Work out the finished part from the listing and answer in its coordinate system (mm). A direction names the side the tool comes from. Give positions to 0.01 mm unless a question says otherwise; leave off trailing zeros. Loops run counter-clockwise (first coordinate to the right, second up) from the corner with the lowest first, then second, coordinate; pieces in that order, holes last. Notation, with made-up numbers: M 5,82 L 54,82 A16 cw 54,94 Z; hole C 8.5,38.25 d6. An arc over 180 degrees is marked long. Write item = value, one per line. Start each with the question number.
1. Consider L1, parallel to X at y = 8.4, z = 25; L2, parallel to X at y = 5.25, z = -35.5; L3, parallel to Y at x = 48.5, z = -9.5. Determine where each line is inside the solid, lowest interval first. Write a range as [from, to].
2. Flat-ended cylindrical pins translate along their axes: pin 1 Ø0.6 at (x, z) = (0.5, -70) entering from +Y; pin 2 Ø1.5 at (x, z) = (-37, 10) entering from -Y; pin 3 Ø6 at (x, y) = (54.5, 0.5) entering from +Z; pin 4 Ø6 at (x, z) = (-55, 0) entering from +Y. Find the tip coordinate at first contact, or state that the pin passes through.
3. Section A-A on y = -5 is taken. Determine the outline of the cut face in (x, z), plus the area to 3 significant figures.
4. The mould has two halves that part along X. Classify faces 5 (the face through (-1, -6.3, -68.5)), 6 (the face through (-50.043, 7.535, -0.651)), 7 (the face through (1, -6.3, 68.6)): released by +X, released by -X, zero draft, split by the parting line, or undercut.
5. For faces 1 (the face through (1, -6.3, -68.5)), 2 (the face through (-1.915, 7.535, 50.669)), 3 (the face through (-1, 5, -1)), 4 (the face through (-1, -6.3, 68.6)), determine the directions among +Z, -Z, +X, -X, +Y, -Y from which every point of the face is accessible in a straight line to the end or side of a thin tool.
6. Section B-B on x = 20 is taken. Give the number of separate pieces and of enclosed holes in the cut face, plus the area to 3 significant figures.
7. Section C-C on y = 2.75 is taken. Determine the outline of the cut face in (x, z), plus the area to 3 significant figures.
```python
from build123d import *

# Parameters (mm, degrees)
SKETCH1_R           = 71.05
BOSS_EXTRUDE1_DEPTH = 10
BOSS_EXTRUDE1_TAPER = 5
SHELL4_T            = -5
SKETCH2_R           = 5
SKETCH2_R_2         = 25
SKETCH2_R_3         = 2.413
CUT_EXTRUDE1_DEPTH  = 101.976259737
CUT_EXTRUDE4_DEPTH  = 10
FILLET2_R           = 5
SKETCH11_R          = 5
CUT_EXTRUDE8_DEPTH  = 101.976259737
SKETCH12_W          = 2
SKETCH12_H          = 2
BOSS_EXTRUDE4_DEPTH = 7.5
SKETCH13_W          = 2
SKETCH13_H          = 4
BOSS_EXTRUDE5_DEPTH = 3
CUT_EXTRUDE9_DEPTH  = 3
CUT_EXTRUDE10_DEPTH = 3
CUT_EXTRUDE11_DEPTH = 3
CUT_EXTRUDE12_DEPTH = 3
CUT_EXTRUDE13_DEPTH = 3
CUT_EXTRUDE14_DEPTH = 3


with BuildPart() as part:
    # Sketch1 → Boss-Extrude1 (new body)
    with BuildSketch(Plane(origin=(0, 0, 0), x_dir=(1, 0, 0), z_dir=(0, 1, 0))):
        Circle(SKETCH1_R)
    extrude(amount=BOSS_EXTRUDE1_DEPTH, taper=BOSS_EXTRUDE1_TAPER)

    # Shell4
    shell4_openings = [part.faces().sort_by_distance(p)[0] for p in [
        (0, 0, 0),
    ]]
    offset(amount=SHELL4_T, openings=shell4_openings, kind=Kind.INTERSECTION)

    # Sketch2 → Cut-Extrude1 (cut, through all)
    with BuildSketch(Plane(origin=(0, 10, 0), x_dir=(1, 0, 0), z_dir=(0, 1, 0))):
        with Locations(Location((0, -46.05, 0), (0, 0, 270))):
            Circle(SKETCH2_R)
        with Locations(Location((0, 36.05, 0), (0, 0, 270))):
            Circle(SKETCH2_R_2)
        with Locations(Location((20, 5, 0), (0, 0, 270))):
            Circle(SKETCH2_R_3)
        with Locations(Location((20, -25, 0), (0, 0, 270))):
            Circle(SKETCH2_R_3)
        with Locations(Location((-20, -25, 0), (0, 0, 270))):
            Circle(SKETCH2_R_3)
        with Locations(Location((-20, 5, 0), (0, 0, 270))):
            Circle(SKETCH2_R_3)
    extrude(amount=-CUT_EXTRUDE1_DEPTH, mode=Mode.SUBTRACT)

    # Sketch6 → Cut-Extrude4 (cut)
    with BuildSketch(Plane(origin=(0, 10, 0), x_dir=(1, 0, 0), z_dir=(0, 1, 0))):
        with BuildLine():
            Line((-2.5, 14.187111582), (2.5, 14.187111582))
            Line((2.5, 14.187111582), (2.5, 9.55))
            ThreePointArc((2.5, 9.55), (2.207106781, 8.842893219), (1.5, 8.55))
            Line((1.5, 8.55), (-1.5, 8.55))
            ThreePointArc((-1.5, 8.55), (-2.207106781, 8.842893219), (-2.5, 9.55))
            Line((-2.5, 9.55), (-2.5, 14.187111582))
        make_face()
    extrude(amount=-CUT_EXTRUDE4_DEPTH, mode=Mode.SUBTRACT)

    # Fillet2
    fillet2_edges = [part.edges().sort_by_distance(p)[0] for p in [
        (-70.175113365, 10, 0),
    ]]
    fillet(fillet2_edges, radius=FILLET2_R)

    # Sketch11 → Cut-Extrude8 (cut, through all)
    with BuildSketch(Plane(origin=(0, 10, 0), x_dir=(1, 0, 0), z_dir=(0, 1, 0))):
        with Locations(Location((-55, 0, 0), (0, 0, 270))):
            Circle(SKETCH11_R)
    extrude(amount=-CUT_EXTRUDE8_DEPTH, mode=Mode.SUBTRACT)

    # Sketch12 → Boss-Extrude4 (add)
    with BuildSketch(Plane(origin=(0, 0, 0), x_dir=(-1, 0, 0), z_dir=(0, -1, 0))):
        Polygon((58.523702054, 32.633974596), (60.255752861, 33.633974596), (59.255752861, 35.366025404), (57.523702054, 34.366025404), align=None)
        with Locations((0, 68)):
            Rectangle(SKETCH12_W, SKETCH12_H)
        Polygon((57.523702054, -34.366025404), (59.255752861, -35.366025404), (60.255752861, -33.633974596), (58.523702054, -32.633974596), align=None)
        with Locations((0, -68)):
            Rectangle(SKETCH12_W, SKETCH12_H)
        Polygon((-58.523702054, -32.633974596), (-60.255752861, -33.633974596), (-59.255752861, -35.366025404), (-57.523702054, -34.366025404), align=None)
        Polygon((-57.523702054, 34.366025404), (-59.255752861, 35.366025404), (-60.255752861, 33.633974596), (-58.523702054, 32.633974596), align=None)
    extrude(amount=BOSS_EXTRUDE4_DEPTH)

    # Sketch13 → Boss-Extrude5 (add)
    with BuildSketch(Plane(origin=(0, -7.5, 0), x_dir=(-1, 0, 0), z_dir=(0, -1, 0))):
        Polygon((-58.523702054, -32.633974596), (-61.987803669, -34.633974596), (-60.987803669, -36.366025404), (-57.523702054, -34.366025404), align=None)
        with Locations((0, -69)):
            Rectangle(SKETCH13_W, SKETCH13_H)
        Polygon((-57.523702054, 34.366025404), (-60.987803669, 36.366025404), (-61.987803669, 34.633974596), (-58.523702054, 32.633974596), align=None)
        with Locations((0, 69)):
            Rectangle(SKETCH13_W, SKETCH13_H)
        Polygon((58.523702054, 32.633974596), (61.987803669, 34.633974596), (60.987803669, 36.366025404), (57.523702054, 34.366025404), align=None)
        Polygon((57.523702054, -34.366025404), (60.987803669, -36.366025404), (61.987803669, -34.633974596), (58.523702054, -32.633974596), align=None)
    extrude(amount=BOSS_EXTRUDE5_DEPTH)

    # Sketch14 → Cut-Extrude9 (cut)
    with BuildSketch(Plane(origin=(1, 0, 0), x_dir=(0, 0, -1), z_dir=(1, 0, 0))):
        Polygon((71, -9), (69, -10.5), (71, -10.5), align=None)
    extrude(amount=-CUT_EXTRUDE9_DEPTH, mode=Mode.SUBTRACT)

    # Sketch16 → Cut-Extrude10 (cut)
    with BuildSketch(Plane(origin=(0.5000000000007515, 0, 0.8660254037857402), x_dir=(0.8660254037844386, 0, -0.4999999999999999), z_dir=(0.49999999999999994, 0, 0.8660254037844387))):
        Polygon((71, -9), (69, -10.5), (71, -10.5), align=None)
    extrude(amount=-CUT_EXTRUDE10_DEPTH, mode=Mode.SUBTRACT)

    # Sketch17 → Cut-Extrude11 (cut)
    with BuildSketch(Plane(origin=(-0.5000000000021357, 0, 0.8660254037881377), x_dir=(0.8660254037844386, 0, 0.4999999999999999), z_dir=(-0.49999999999999994, 0, 0.8660254037844387))):
        Polygon((71, -9), (69, -10.5), (71, -10.5), align=None)
    extrude(amount=-CUT_EXTRUDE11_DEPTH, mode=Mode.SUBTRACT)

    # Sketch18 → Cut-Extrude12 (cut)
    with BuildSketch(Plane.ZY.offset(1)):
        Polygon((71, -9), (69, -10.5), (71, -10.5), align=None)
    extrude(amount=-CUT_EXTRUDE12_DEPTH, mode=Mode.SUBTRACT)

    # Sketch19 → Cut-Extrude13 (cut)
    with BuildSketch(Plane(origin=(-0.5000000000020854, 0, -0.8660254037880506), x_dir=(-0.8660254037844386, 0, 0.4999999999999999), z_dir=(-0.49999999999999994, 0, -0.8660254037844387))):
        Polygon((71, -9), (69, -10.5), (71, -10.5), align=None)
    extrude(amount=-CUT_EXTRUDE13_DEPTH, mode=Mode.SUBTRACT)

    # Sketch20 → Cut-Extrude14 (cut)
    with BuildSketch(Plane(origin=(0.5000000000006769, 0, -0.8660254037856109), x_dir=(-0.8660254037844386, 0, -0.4999999999999999), z_dir=(0.49999999999999994, 0, -0.8660254037844387))):
        Polygon((71, -9), (69, -10.5), (71, -10.5), align=None)
    extrude(amount=-CUT_EXTRUDE14_DEPTH, mode=Mode.SUBTRACT)


solid = part.part
```
Verdict:
q1.L1 = [-64.59, -22.41], [-17.59, 17.59], [22.41, 64.59]
q1.L2 = [-61.01, -24.99], [24.99, 61.01]
q1.L3 = [5, 10]
q2.pin_1 = 7.85
q2.pin_2 = 5
q2.pin_3 = 48.91
q2.pin_4 = through
q3.outline = M -60.26,-33.63 L -59.26,-35.37 L -57.52,-34.37 L -58.52,-32.63 Z; M -60.26,33.63 L -58.52,32.63 L -57.52,34.37 L -59.26,35.37 Z; M -1,-69 L 1,-69 L 1,-67 L -1,-67 Z; M -1,67 L 1,67 L 1,69 L -1,69 Z; M 57.52,-34.37 L 59.26,-35.37 L 60.26,-33.63 L 58.52,-32.63 Z; M 57.52,34.37 L 58.52,32.63 L 60.26,33.63 L 59.26,35.37 Z
q3.area = 24.0 mm2
q4.face_5 = released by -X
q4.face_6 = undercut
q4.face_7 = released by +X
q5.face_1 = +Z, -Z, +X, -Y
q5.face_2 = +Y, -Y
q5.face_3 = -Y
q5.face_4 = +Z, -Z, -X, -Y
q6.separate_pieces = 4
q6.enclosed_holes = 0
q6.area = 520 mm2
q7.outline = C 0,0 d141.62; hole C 0,0 d131.58
q7.area = 2,150 mm2
